Verification items for the finished model (mm, model axes). A direction names the side the tool comes from. Round coordinates to 2 decimals unless told otherwise and drop trailing zeros. Loops run counter-clockwise (first coordinate to the right, second up) from the corner with the lowest first, then second, coordinate; pieces in that order, holes last. Notation, with made-up numbers: (75.25, -1.75) - (99.25, -1.75) arc R18 ccw to (99.25, 5.25) - close; hole circle Ø8 at (16, -21.5). An arc over 180 degrees is marked (long way). Use CSV: the item, a comma, the result in double quotes.
```python
from build123d import *

# Parameters (mm, degrees)
F1_DEPTH = 18.25625
F3_DEPTH = 609.6
F4_DEPTH = 609.6


with BuildPart() as f1:
    # F0 (on Top) → F1 (new body)
    with BuildSketch(Plane.XY):
        Polygon((609.6, 263.398), (609.6, 304.8), (-609.6, 304.8), (-609.6, -134.874), (0, -134.874), (0, -263.398), (-609.6, -263.398), (-609.6, -304.8), (609.6, -304.8), (609.6, 134.874), (0, 134.874), (0, 263.398), align=None)
    extrude(amount=-F1_DEPTH)

    # F2 (on Right) → F3 (join, through all)
    with BuildSketch(Plane.YZ):
        Polygon((65.5882849274, 27.5459089179), (263.398, 55.3462513865), (281.65425, 57.912), (279.1134710756, 75.99058143), (0, 36.7637412283), align=None)
        Polygon((263.398, 55.3462513865), (263.398, 0), (281.65425, 0), (281.65425, 57.912), align=None)
        Polygon((0, 18.3280766075), (65.5882849274, 27.5459089179), (0, 36.7637412283), (-65.5882849274, 27.5459089179), align=None)
        Polygon((-259.0468322931, -18.07858143), (0, 18.3280766075), (-65.5882849274, 27.5459089179), (-261.5876112175, 0), align=None)
    extrude(amount=-F3_DEPTH)

    # F2 (on Right) → F4 (join, through all)
    with BuildSketch(Plane.YZ):
        Polygon((-263.398, 0), (-263.398, 55.3462513865), (-281.65425, 57.912), (-281.65425, 0), align=None)
        Polygon((-65.5882849274, 27.5459089179), (0, 36.7637412283), (-279.1134710756, 75.99058143), (-281.65425, 57.912), (-263.398, 55.3462513865), align=None)
        Polygon((0, 18.3280766075), (65.5882849274, 27.5459089179), (0, 36.7637412283), (-65.5882849274, 27.5459089179), align=None)
        Polygon((261.5876112175, 0), (65.5882849274, 27.5459089179), (0, 18.3280766075), (259.0468322931, -18.07858143), align=None)
    extrude(amount=F4_DEPTH)


solid = f1.part
```
1) Cross-section at B-B, the plane y = -106. Record the cut outline in (x, z), then the cut area to 3 significant figures.
Returned:
outline,"(-609.6, -18.26) - (609.6, -18.26) - (609.6, 0) - (-609.6, 0) - close; (-609.6, 3.43) - (0, 3.43) - (0, 21.87) - (-609.6, 21.87) - close; (0, 33.23) - (609.6, 33.23) - (609.6, 51.66) - (0, 51.66) - close"
area,"44,700 mm²"
2) Cross-section at C-C, the plane y = 191. Record the cut outline in (x, z), then the cut area to 3 significant figures.
Returned:
outline,"(-609.6, -18.26) - (0, -18.26) - (0, -8.52) - (609.6, -8.52) - (609.6, 9.92) - (0, 9.92) - (0, 0) - (-609.6, 0) - close; (-609.6, 45.17) - (0, 45.17) - (0, 63.61) - (-609.6, 63.61) - close"
area,"33,600 mm²"
3) Cross-section at A-A, the plane x = -382. Record the cut outline in (y, z).
Returned:
outline,"(-304.8, -18.26) - (-263.4, -18.26) - (-263.4, 0) - (-304.8, 0) - close; (-261.59, 0) - (-259.05, -18.08) - (-134.87, -0.63) - (-134.87, -18.26) - (304.8, -18.26) - (304.8, 0) - (281.65, 0) - (281.65, 57.91) - (279.11, 75.99) - close; hole (-130.41, 0) - (263.4, 0) - (263.4, 55.35) - close"
4) Gauge pin test, flat ends, axial feed: pin 1 Ø12.5 at (x, y) = (269.5, 281) entering from +Z; pin 2 Ø2 at (x, z) = (405, 45.5) entering from -Y; pin 3 Ø12 at (x, y) = (-205, -174.5) entering from +Z. Record the tip position at first contact, or that the pin passes through.
Returned:
pin 1,"stops at z = 0"
pin 2,"stops at y = -281.65"
pin 3,"stops at z = 13.08"
5) Mould release check, pull along Y, two halves, no side actions. Record for faces 6 (the face through (300.53, -69.25, 28.06)), 7 (the face through (-609.6, 81, -2)), 8 (the face through (-300.533, 12.548, 38.527)), 9 (the face through (0, 129, 11)): +Y half, -Y half, draft (parallel to the pull), parting line (faces both ways), or undercut.
Returned:
face 6,"undercut"
face 7,"draft"
face 8,"-Y half"
face 9,"undercut"
6) Access from +Z, -Z, +X, -X, +Y, -Y to the whole of each face (thin tool, end or side, straight path). Record for faces 1 (the face through (301, -263.398, 27)), 2 (the face through (-301, 281.654, 29)), 3 (the face through (0, 182, 49)), 4 (the face through (0, -133, 11)), 5 (the face through (300.53, 196.09, -9.23)).
Returned:
face 1,"+X, -X"
face 2,"+Z, +X, -X, +Y"
face 3,"+Z, +X, +Y"
face 4,"+X"
face 5,"-Z, +X"
7) Thickness scan on probe 1 along Z at (x, y) = (226, -71); probe 2 along X at (y, z) = (-145, 44); probe 3 along Z at (x, y) = (381, -191). Record the ranges inside material, lowest first. Write a range as [from, to].
Returned:
probe 1,"z = [-18.26, 0], [28.31, 46.74]"
probe 2,"x = [0, 609.6]"
probe 3,"z = [-18.26, 0], [45.17, 63.61]"
